Geometry: final body of the model. Coordinates: model frame, mm. Coordinates: 2 decimals unless noted, no trailing zeros. Order: outer loops, then holes, each group sorted by start corner. A loop starts at its lowest first (then second) coordinate and runs counter-clockwise, first axis right, second up. Notation, with made-up numbers: (-24.75, 22.5) -> (15.25, 22.5) arc R10 cw to (15.25, 39.5) -> close; hole circle Ø5 at (22.5, 66.5). An arc over 180 degrees is marked (long way). Use one line per item in the form item = value.
```python
from build123d import *

# Parameters (mm, degrees)
F0_R     = 20.32
F0_R_2   = 0.9525
F1_DEPTH = 2.54
F2_R     = 5.08


with BuildPart() as f1:
    # F0 (on Top) → F1 (new body)
    with BuildSketch(Plane.XY):
        with BuildLine():
            ThreePointArc((2.5368230131, 25.273), (0, 27.94), (-2.5368230131, 25.273))
            ThreePointArc((-2.5368230131, 25.273), (0, -25.4), (2.5368230131, 25.273))
        make_face()
        Circle(F0_R, mode=Mode.SUBTRACT)
        with Locations((0, 25.4)):
            Circle(F0_R_2, mode=Mode.SUBTRACT)
    extrude(amount=F1_DEPTH)

    # F2
    f2_edges = [f1.edges().sort_by_distance(p)[0] for p in [
        (-2.536823, 25.273, 1.27),
        (2.536823, 25.273, 1.27),
    ]]
    fillet(f2_edges, radius=F2_R)


solid = f1.part
```
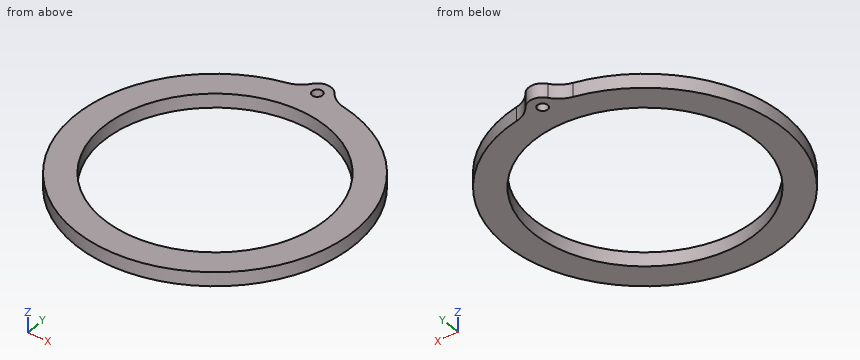
1) Section A-A, the plane x = 0. Output: boundary loops of the cut face in (y, z), and give its area (3 significant figures).
Results found:
outline = (-25.4, 0) -> (-20.32, 0) -> (-20.32, 2.54) -> (-25.4, 2.54) -> close; (20.32, 0) -> (24.45, 0) -> (24.45, 2.54) -> (20.32, 2.54) -> close; (26.35, 0) -> (27.94, 0) -> (27.94, 2.54) -> (26.35, 2.54) -> close
area = 27.4 mm2
2) Section C-C, the plane x = -19.5. Output: boundary loops of the cut face in (y, z).
Results found:
outline = (-16.28, 0) -> (-5.71, 0) -> (-5.71, 2.54) -> (-16.28, 2.54) -> close; (5.71, 0) -> (16.28, 0) -> (16.28, 2.54) -> (5.71, 2.54) -> close
3) Section D-D, the plane z = 0.5. Give the number of separate pieces and of enclosed holes in the cut face, and give its area (3 significant figures).
Results found:
separate_pieces = 1
enclosed_holes = 2
area = 739 mm2
4) Section B-B, the plane y = 6. Output: boundary loops of the cut face in (x, z).
Results found:
outline = (-24.68, 0) -> (-19.41, 0) -> (-19.41, 2.54) -> (-24.68, 2.54) -> close; (19.41, 0) -> (24.68, 0) -> (24.68, 2.54) -> (19.41, 2.54) -> close
5) Material intervals for probe 1 along Y at (x, z) = (0, 0.55); probe 2 along Y at (x, z) = (4, 0.55); probe 3 along Y at (x, z) = (-2, 1.65), sorted ascending. Write a range as from..to.
Results found:
probe_1 = -25.4..-20.32, 20.32..24.45, 26.35..27.94
probe_2 = -25.08..-19.92, 19.92..25.26
probe_3 = -25.32..-20.22, 20.22..26.97
